```python
from build123d import *

# Parameters (mm, degrees)
SKETCH1_R           = 17.5
SKETCH1_R_2         = 1.5
BOSS_EXTRUDE1_DEPTH = 1.5
CHAMFER1_SIZE       = 0.2


with BuildPart() as part:
    # Sketch1 → Boss-Extrude1 (new body)
    with BuildSketch(Plane.XY):
        Circle(SKETCH1_R)
        with Locations((-8, 9)):
            Circle(SKETCH1_R_2, mode=Mode.SUBTRACT)
        with Locations((8, 9)):
            Circle(SKETCH1_R_2, mode=Mode.SUBTRACT)
        with BuildLine():
            Line((8.337397166, -2.5), (6.837397166, -2.5))
            ThreePointArc((6.837397166, -2.5), (-7, -4), (6.837397166, -5.5))
            Line((6.837397166, -5.5), (8.337397166, -5.5))
            Line((8.337397166, -5.5), (8.337397166, -2.5))
        make_face(mode=Mode.SUBTRACT)
    extrude(amount=BOSS_EXTRUDE1_DEPTH)

    # Chamfer1
    chamfer1_edges = [part.edges().sort_by_distance(p)[0] for p in [
        (-7, -4, 1.5),
        (7.587397166, -5.5, 1.5),
        (6.5, 9, 0),
        (6.5, 9, 1.5),
        (-17.5, 0, 0),
        (-9.5, 9, 0),
        (-9.5, 9, 1.5),
        (-17.5, 0, 1.5),
        (8.337397166, -4, 0),
        (7.587397166, -2.5, 0),
        (-7, -4, 0),
        (7.587397166, -5.5, 0),
        (8.337397166, -4, 1.5),
        (7.587397166, -2.5, 1.5),
    ]]
    chamfer(chamfer1_edges, length=CHAMFER1_SIZE)


solid = part.part
```
The model under review builds one solid part; all positions refer to its coordinate system, in mm. A direction names the side the tool comes from. Round coordinates to 2 decimals unless told otherwise and drop trailing zeros. Order: outer loops, then holes, each group sorted by start corner. A loop starts at its lowest first (then second) coordinate and runs counter-clockwise, first axis right, second up. Notation, with made-up numbers: (55, 15.5) - (94, 15.5) arc R23 cw to (94, 46.5) - close; hole circle Ø11 at (13, 37). An arc over 180 degrees is marked (long way). Answer in a Markdown table with one row per item.
(1) Take a section at B-B on z = 0.95. Write out the cut boundary in (x, y), plus the area to 3 significant figures.
Result set:
| item | result |
|---|---|
| outline | circle Ø35 at (0, 0); hole circle Ø3 at (-8, 9); hole circle Ø3 at (8, 9); hole (6.84, -5.5) - (8.34, -5.5) - (8.34, -2.5) - (6.84, -2.5) arc R7 ccw (long way) to start |
| area | 790 mm2 |
(2) Machinability: for faces 1 (the face through (8.337, -4, 1)), 2 (the face through (0, 4, 0)), which of the approach directions +Z, -Z, +X, -X, +Y, -Y give a long, thin tool a straight path to every point of the face, cutting with its end or side? Answer none if there is none.
Result set:
| item | result |
|---|---|
| face 1 | +Z, -Z |
| face 2 | -Z, +X, -X, +Y, -Y |
(3) Take a section at A-A on x = 0. Write out the cut boundary in (y, z), plus the area to 3 significant figures.
Result set:
| item | result |
|---|---|
| outline | (-17.5, 0.2) - (-17.3, 0) - (-11.2, 0) - (-11, 0.2) - (-11, 1.3) - (-11.2, 1.5) - (-17.3, 1.5) - (-17.5, 1.3) - close; (3, 0.2) - (3.2, 0) - (17.3, 0) - (17.5, 0.2) - (17.5, 1.3) - (17.3, 1.5) - (3.2, 1.5) - (3, 1.3) - close |
| area | 31.3 mm2 |
(4) Clearance check with flat-ended pins moving along their axes: P1, Ø0.6, axis at x = 7.5, z = 0.5, coming from the +Y side; P2, Ø18, axis at x = 0, y = -4, coming from the -Z side; P3, Ø0.9, axis at y = -4.5, z = 1, coming from the -X side. State where each tip first meets the part, or that it passes through.
Result set:
| item | result |
|---|---|
| P1 | stops at y = 15.95 |
| P2 | stops at z = 0 |
| P3 | stops at x = -17.02 |
(5) Take a section at C-C on y = 9. Count the separate pieces of the cut face and the enclosed holes in it, plus the area to 3 significant figures.
Result set:
| item | result |
|---|---|
| separate pieces | 3 |
| enclosed holes | 0 |
| area | 35.8 mm2 |
(6) For line 1 (Y direction, x = 0, z = 0.8); line 2 (Y direction, x = 8, z = 1.05); line 3 (Y direction, x = -3.5, z = 1.3), list the stretches that pass through material, from the lowest coordinate up. Write a range as from..to.
Result set:
| item | result |
|---|---|
| line 1 | y = -17.5..-11, 3..17.5 |
| line 2 | y = -15.56..-5.5, -2.5..7.5, 10.5..15.56 |
| line 3 | y = -17.15..-10.06, 2.06..17.15 |
(7) Mouldability with a two-part tool opening along Y and no side actions: class faces 3 (the face through (0, 4, 1.5)), 4 (the face through (-13.887, -10.648, 0.742)), 5 (the face through (-9.2, 8.1, 0.7)) as released by +Y, released by -Y, zero draft, split by the parting line, or undercut.
Result set:
| item | result |
|---|---|
| face 3 | zero draft |
| face 4 | split by the parting line |
| face 5 | undercut |
